from build123d import *

# Parameters (mm, degrees)
SKETCH2_R           = 5
BOSS_EXTRUDE1_DEPTH = 6
BOSS_EXTRUDE2_START = -14
SKETCH3_R           = 5
BOSS_EXTRUDE2_DEPTH = 14


with BuildPart() as part:
    # Sketch2 → Boss-Extrude1 (new body)
    with BuildSketch(Plane(origin=(0, 0, 0), x_dir=(1, 0, 0), z_dir=(0, 1, 0))):
        with BuildLine():
            Line((13.274432238, 35.765352266), (13.274432238, -125.251116332))
            Line((13.274432238, -125.251116332), (13.274432238, -154.229901261))
            Line((13.274432238, -154.229901261), (0.452829748, -154.229901261))
            Line((0.452829748, -154.229901261), (0.452829748, -125.251116332))
            Line((0.452829748, -125.251116332), (0.452829748, 35.765352266))
            ThreePointArc((0.452829748, 35.765352266), (6.863630993, 78.970129688), (13.274432238, 35.765352266))
        make_face()
        with Locations(Location((6.863630993, 56.892117967, 0), (0, 0, 90))):
            Circle(SKETCH2_R, mode=Mode.SUBTRACT)
        with Locations(Location((6.863630993, -146.377882033, 0), (0, 0, 270))):
            Circle(SKETCH2_R, mode=Mode.SUBTRACT)
    extrude(amount=BOSS_EXTRUDE1_DEPTH)

    # Sketch3 → Boss-Extrude2 (add)
    with BuildSketch(Plane(origin=(0, 6, 0), x_dir=(1, 0, 0), z_dir=(0, 1, 0)).offset(BOSS_EXTRUDE2_START)):
        with Locations(Location((6.863630993, 56.892117967, 0), (0, 0, 270))):
            Circle(SKETCH3_R)
    extrude(amount=BOSS_EXTRUDE2_DEPTH)


solid = part.part
Geometry check sheet. Reference: the model listing, model coordinates, mm. A direction names the side the tool comes from. Coordinates: 2 decimals unless noted, no trailing zeros. Order: outer loops, then holes, each group sorted by start corner. A loop starts at its lowest first (then second) coordinate and runs counter-clockwise, first axis right, second up. Notation, with made-up numbers: (49, -11.5) -> (56, -11.5) arc R29 cw to (56, 21.5) -> close; hole circle Ø1 at (2.5, 14). An arc over 180 degrees is marked (long way). Use a Markdown table: item, result. Add a question column.
1. Material ranges on L1, parallel to Y at x = 2, z = 18.5; L2, parallel to X at y = 1.25, z = 105; L3, parallel to Z at x = 10.5, y = 1.5, recorded low to high.
2. Cross-section at D-D (x = -5). Enter the section's corners in (y, z), and give its area (3 significant figures).
3. Set-up check for faces 1 (the face through (7, 6, 10)), 2 (the face through (13.274, 3, 58)), 3 (the face through (8.365, -4.056, -52.123)), 4 (the face through (0.453, 3, 61)): record each of +Z, -Z, +X, -X, +Y, -Y from which the full face is reachable in a straight line by a thin tool's end or side.
4. Cross-section at A-A (x = 9). Enter the section's corners in (y, z), and give its area (3 significant figures).
5. Cross-section at C-C (y = -6). Enter the section's corners in (x, z).
6. Cross-section at B-B (z = -59.5). Enter the section's corners in (x, y).
7. Mould release check, pull along Z, two halves, no side actions. Record for faces 5 (the face through (8.365, 2.958, 151.147)), 6 (the face through (7, 3, 154.23)), 7 (the face through (7, -8, -57)), 8 (the face through (5.984, 2.958, -78.953)): pulls with the +Z half, pulls with the -Z half, needs draft (parallel to the pull), parting line crosses it, or undercut.
8. Go/stop test with flat-tipped pins: pin 1 Ø5 at (y, z) = (3, 23.5) entering from +X; pin 2 Ø6 at (x, z) = (6.86, 146.38) entering from +Y; pin 3 Ø13 at (x, z) = (8, 14.5) entering from -Y; pin 4 Ø5 at (y, z) = (2, 65) entering from -X. Record where each tip stops, or that it passes through.
Filled sheet:
| question | item | result |
|---|---|---|
| 1 | L1 | 0 to 6 |
| 1 | L2 | 0.45 to 13.27 |
| 1 | L3 | -78.67 to 142.95, 149.81 to 154.23 |
| 2 | outline | (0, -75.51) -> (6, -75.51) -> (6, -38.27) -> (0, -38.27) -> close |
| 2 | area | 223 mm2 |
| 3 | face 1 | +Z, -Z, +X, -X, +Y |
| 3 | face 2 | +Z, +X, +Y, -Y |
| 3 | face 3 | -Y |
| 3 | face 4 | +Z, -X, +Y, -Y |
| 4 | outline | (-8, -61.41) -> (0, -61.41) -> (0, -78.87) -> (6, -78.87) -> (6, 141.86) -> (0, 141.86) -> (0, -52.37) -> (-8, -52.37) -> close; (0, 150.9) -> (6, 150.9) -> (6, 154.23) -> (0, 154.23) -> close |
| 4 | area | 1,420 mm2 |
| 5 | outline | circle Ø10 at (6.86, -56.89) |
| 6 | outline | (-15.06, 0) -> (2.6, 0) -> (2.6, -8) -> (11.13, -8) -> (11.13, 0) -> (28.79, 0) -> (28.79, 6) -> (-15.06, 6) -> close |
| 7 | face 5 | undercut |
| 7 | face 6 | pulls with the +Z half |
| 7 | face 7 | needs draft |
| 7 | face 8 | parting line crosses it |
| 8 | pin 1 | x = 13.27 |
| 8 | pin 2 | through |
| 8 | pin 3 | y = 0 |
| 8 | pin 4 | x = 0.45 |
